Read the model definition and answer for the solid it produces. Units are mm, in the model's axes. A direction names the side the tool comes from. Coordinates: 2 decimals unless noted, no trailing zeros. Loops run counter-clockwise (first coordinate to the right, second up) from the corner with the lowest first, then second, coordinate; pieces in that order, holes last. Notation, with made-up numbers: M 83.25,-37.75 L 137.25,-37.75 A30 cw 137.25,-10.75 Z; hole C 38,81.25 d11. An arc over 180 degrees is marked long. Put each result on its own line as item: value.
from build123d import *

# Parameters (mm, degrees)
SKETCH1_R           = 2
BOSS_EXTRUDE1_DEPTH = 5
SKETCH2_R           = 5
CUT_EXTRUDE1_DEPTH  = 3.5
SKETCH3_R           = 1
CUT_EXTRUDE2_DEPTH  = 2
CHAMFER1_SIZE       = 1.5


with BuildPart() as part:
    # Sketch1 → Boss-Extrude1 (new body)
    with BuildSketch(Plane.XY):
        with BuildLine():
            Line((0, -6.5), (-13.5, -6.5))
            Line((-13.5, -6.5), (-13.5, 8.5))
            Line((-13.5, 8.5), (-11.5, 8.5))
            Line((-11.5, 8.5), (1.065452768, 6.412083156))
            ThreePointArc((1.065452768, 6.412083156), (6.477983502, -0.534536942), (0, -6.5))
        make_face()
        Circle(SKETCH1_R, mode=Mode.SUBTRACT)
    extrude(amount=BOSS_EXTRUDE1_DEPTH)

    # Sketch2 → Cut-Extrude1 (cut)
    with BuildSketch(Plane.XY.offset(5)):
        Circle(SKETCH2_R)
    extrude(amount=-CUT_EXTRUDE1_DEPTH, mode=Mode.SUBTRACT)

    # Sketch3 → Cut-Extrude2 (cut)
    with BuildSketch(Plane.ZY.offset(13.5)):
        with Locations(Location((2.5, 6, 0), (0, 0, 270))):
            Circle(SKETCH3_R)
        with Locations(Location((2.5, -4, 0), (0, 0, 90))):
            Circle(SKETCH3_R)
    extrude(amount=-CUT_EXTRUDE2_DEPTH, mode=Mode.SUBTRACT)

    # Chamfer1
    chamfer1_edges = [part.edges().sort_by_distance(p)[0] for p in [
        (-5.217273616, 7.456041578, 0),
        (6.477983502, -0.534536942, 0),
        (-6.75, -6.5, 0),
    ]]
    chamfer(chamfer1_edges, length=CHAMFER1_SIZE)


solid = part.part
1) Find section C-C, the plane x = -8.75. Write down the section's boundary in (y, z).
Answer list:
outline: M -6.5,1.5 L -5,0 L 6.52,0 L 8.04,1.5 L 8.04,5 L -6.5,5 Z
2) Find section A-A, the plane y = 0. Write down the section's boundary in (x, z).
Answer list:
outline: M -13.5,0 L -2,0 L -2,1.5 L -5,1.5 L -5,5 L -13.5,5 Z; M 2,0 L 5,0 L 6.5,1.5 L 6.5,5 L 5,5 L 5,1.5 L 2,1.5 Z
3) Determine the mould class of faces 1 (the conical face through (5.25, -0.32, 0.26)), 2 (the flat face through (-0.1, -2.2, 1.5)), 3 (the flat face through (-7, -6.5, 3)) for opening direction X: released by +X, released by -X, zero draft, split by the parting line, or undercut.
Answer list:
face 1: released by +X
face 2: undercut
face 3: zero draft
4) Straight lines are drawn through the part: line 1 (Z direction, x = -11.75, y = -4); line 2 (Z direction, x = 0.25, y = 3.5); line 3 (Y direction, x = 1.75, z = 4.7). For each, find the intervals that lie inside material, in ascending order. Write a range as [from, to].
Answer list:
line 1: z = [0, 1.5], [3.5, 5]
line 2: z = [0, 1.5]
line 3: y = [-6.26, -4.68], [4.68, 6.26]
5) Find section D-D, the plane z = 4.3. Write down the section's boundary in (x, y).
Answer list:
outline: M -13.5,-6.5 L 0,-6.5 A6.5 ccw 1.07,6.41 L -11.5,8.5 L -13.5,8.5 Z; hole C 0,0 d10
6) Find section B-B, the plane z = 2.5. Write down the section's boundary in (x, y).
Answer list:
outline: M -13.5,-6.5 L 0,-6.5 A6.5 ccw 1.07,6.41 L -11.5,8.5 L -13.5,8.5 L -13.5,7 L -11.5,7 L -11.5,5 L -13.5,5 L -13.5,-3 L -11.5,-3 L -11.5,-5 L -13.5,-5 Z; hole C 0,0 d10
7) Which of the six approach directions +Z, -Z, +X, -X, +Y, -Y give full straight-line access (tool end or side, diameter ignored) to faces 4 (the cylindrical face through (-1.08, -4.88, 3.27)), 5 (the flat face through (-6, 1, 5)), 6 (the cylindrical face through (-12.5, -4.8, 3.1))?
Answer list:
face 4: +Z
face 5: +Z, +X, -X, +Y, -Y
face 6: -X
8) Given pin 1 Ø1.8 at (y, z) = (-4, 2.5) entering from +X; pin 2 Ø1.6 at (y, z) = (-4, 2.5) entering from -X; pin 3 Ø3 at (y, z) = (6, 2.5) entering from +X; pin 4 Ø1 at (x, y) = (-4, 6) entering from -Z, each flat-ended and moving along its own axis, determine where each tip first touches the part or whether it passes through.
Answer list:
pin 1: stops at x = 5.71
pin 2: stops at x = -11.5
pin 3: stops at x = 4.69
pin 4: stops at z = 0
